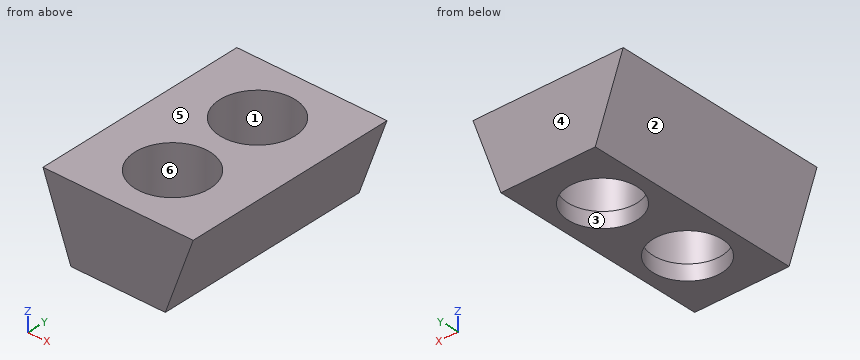
from build123d import *

# Parameters (mm, degrees)
SKETCH1_W           = 12.446
SKETCH1_H           = 18.0975
SKETCH1_R           = 3.1115
BOSS_EXTRUDE1_DEPTH = 6.35
CUT_EXTRUDE1_DEPTH  = 23.863615686
SKETCH3_R           = 3.1115
SKETCH3_R_2         = 2.8575
BOSS_EXTRUDE2_DEPTH = 1.27


with BuildPart() as part:
    # sketch1 → Boss-Extrude1 (new body)
    with BuildSketch(Plane.XY):
        with Locations((6.223, 9.04875)):
            Rectangle(SKETCH1_W, SKETCH1_H)
        with Locations((6.223, 5.08)):
            Circle(SKETCH1_R, mode=Mode.SUBTRACT)
        with Locations((6.223, 13.0175)):
            Circle(SKETCH1_R, mode=Mode.SUBTRACT)
    extrude(amount=BOSS_EXTRUDE1_DEPTH)

    # Sketch2 → Cut-Extrude1 (cut, through all)
    with BuildSketch(Plane(origin=(0, 18.0975, 0), x_dir=(1, 0, 0), z_dir=(0, 1, 0))):
        Polygon((0, -6.35), (0, 0), (2.311210988, 0), align=None)
        Polygon((12.446, -6.35), (12.446, 0), (10.134789012, 0), align=None)
    extrude(amount=-CUT_EXTRUDE1_DEPTH, mode=Mode.SUBTRACT)

    # Sketch3 → Boss-Extrude2 (add)
    # profile 1 of 2: a face of its own
    with BuildSketch(Plane(origin=(0, 0, 0), x_dir=(-1, 0, 0), z_dir=(0, 0, -1))):
        with Locations((-6.223, 5.08)):
            Circle(SKETCH3_R)
        with Locations((-6.223, 5.08)):
            Circle(SKETCH3_R_2, mode=Mode.SUBTRACT)
    # profile 2 of 2: a face of its own
    with BuildSketch(Plane(origin=(0, 0, 0), x_dir=(-1, 0, 0), z_dir=(0, 0, -1))):
        with Locations((-6.223, 13.0175)):
            Circle(SKETCH3_R)
        with Locations((-6.223, 13.0175)):
            Circle(SKETCH3_R_2, mode=Mode.SUBTRACT)
    extrude(amount=-BOSS_EXTRUDE2_DEPTH)


solid = part.part
Verification items for the finished model (mm, model axes). Face numbers are marked on the shaded views. A direction names the side the tool comes from. Give positions to 0.01 mm unless a question says otherwise; leave off trailing zeros. Write each loop counter-clockwise with the first axis right and the second up, starting at its lowest first coordinate (ties: lowest second). Pieces come first, ordered by that corner, then holes. Notation, with made-up numbers: (62.25, 61.25) - (83.25, 61.25) arc R36 ccw to (83.25, 99.25) - close; hole circle Ø10 at (-24.75, -13.5). An arc over 180 degrees is marked (long way). Answer as CSV lines item,"result". Start each with the question number.
1. Thickness scan on line 1 (Y direction, x = 5, z = 4.5); line 2 (Y direction, x = 8, z = 6); line 3 (X direction, y = 6.75, z = 3.25). Record the ranges inside material, lowest first.
2. Sectioned sample at A-A (y = 5.08). Record the boundary of the cut face in (x, z), then the cut area to 3 significant figures.
3. Set-up check for the marked faces 5 and 6: record each of +Z, -Z, +X, -X, +Y, -Y from which the full face is reachable in a straight line by a thin tool's end or side.
4. Depth check by flat-ended pin: pin 1 (1 mm diameter, centred on y = 14, z = 2.5, fed in from -X); pin 2 (7 mm diameter, centred on x = 6.223, y = 5.08, fed in from +Z); pin 3 (1.5 mm diameter, centred on y = 9.5, z = 5.5, fed in from -X). Enter the tip coordinate at first touch or a pass-through.
5. Draft check along Y on the marked faces 1, 2, 3 and 4. Enter one of: pulls with the +Y half, pulls with the -Y half, needs draft (parallel to the pull), parting line crosses it, or undercut.
6. Sectioned sample at C-C (z = 3). Record the boundary of the cut face in (x, y).
7. Sectioned sample at D-D (x = 4). Record the boundary of the cut face in (y, z).
8. Sectioned sample at B-B (x = 7.25). Record the boundary of the cut face in (y, z), then the cut area to 3 significant figures.
Derived:
1,line 1,"0 to 2.22, 7.94 to 10.16, 15.88 to 18.1"
1,line 2,"0 to 2.53, 7.63 to 10.46, 15.57 to 18.1"
1,line 3,"1.13 to 3.6, 8.85 to 11.32"
2,outline,"(0, 6.35) - (2.31, 0) - (3.37, 0) - (3.37, 1.27) - (3.11, 1.27) - (3.11, 6.35) - close; (9.08, 0) - (10.13, 0) - (12.45, 6.35) - (9.33, 6.35) - (9.33, 1.27) - (9.08, 1.27) - close"
2,area,"25.5 mm²"
3,face 5,"+Z, +X, -X, +Y, -Y"
3,face 6,"+Z"
4,pin 1,"x = 1.22"
4,pin 2,"z = 6.35"
4,pin 3,"x = 0.04"
5,face 1,"undercut"
5,face 2,"needs draft"
5,face 3,"undercut"
5,face 4,"pulls with the +Y half"
6,outline,"(1.22, 0) - (11.23, 0) - (11.23, 18.1) - (1.22, 18.1) - close; hole circle Ø6.22 at (6.22, 5.08); hole circle Ø6.22 at (6.22, 13.02)"
7,outline,"(0, 0) - (3.28, 0) - (3.28, 1.27) - (2.9, 1.27) - (2.9, 6.35) - (0, 6.35) - close; (6.88, 0) - (11.22, 0) - (11.22, 1.27) - (10.84, 1.27) - (10.84, 6.35) - (7.26, 6.35) - (7.26, 1.27) - (6.88, 1.27) - close; (14.81, 0) - (18.1, 0) - (18.1, 6.35) - (15.19, 6.35) - (15.19, 1.27) - (14.81, 1.27) - close"
8,outline,"(0, 0) - (2.41, 0) - (2.41, 1.27) - (2.14, 1.27) - (2.14, 6.35) - (0, 6.35) - close; (7.75, 0) - (10.35, 0) - (10.35, 1.27) - (10.08, 1.27) - (10.08, 6.35) - (8.02, 6.35) - (8.02, 1.27) - (7.75, 1.27) - close; (15.68, 0) - (18.1, 0) - (18.1, 6.35) - (15.95, 6.35) - (15.95, 1.27) - (15.68, 1.27) - close"
8,area,"41.7 mm²"
